Could you check a few things on this model? Use its own coordinates, in mm. A direction names the side the tool comes from. Coordinates: 2 decimals unless noted, no trailing zeros. Order: outer loops, then holes, each group sorted by start corner. A loop starts at its lowest first (then second) coordinate and runs counter-clockwise, first axis right, second up. Notation, with made-up numbers: (68, 9) - (118, 9) arc R24 ccw to (118, 44) - close; hole circle Ø3 at (17, 39). An arc over 180 degrees is marked (long way). Answer as a JSON object with one key per item and string values. Group by question number.
(1) Imagine slicing it at D-D, the plane x = 2.25. Write out the boundary of the cut face in (y, z), and give its area (3 significant figures).
(2) Please list where these lines run through material, in increasing order: probe 1 along Y at (x, z) = (8, 0); probe 2 along Z at (x, y) = (4, 0.2); probe 3 along X at (y, z) = (-0.85, 1.15).
(3) Imagine slicing it at C-C, the plane x = 0.75. Write out the boundary of the cut face in (y, z), and give its area (3 significant figures).
(4) Will these pins go through, and if not, where does the flat tip stop? P1, Ø0.5, axis at x = -1, y = 0, coming from the -Z side; P2, Ø1, axis at x = 1, y = 1, coming from the -Z side; P3, Ø1.5, axis at y = 0, z = 0.5, coming from the -X side; P4, Ø2, axis at x = 8.5, y = -1, coming from the +Z side.
(5) Which directions (+Z, -Z, +X, -X, +Y, -Y) give clear straight access to the entire face, cutting with the end or side of a thin tool? Please do faces 1 (the cylindrical face through (0.61, 0.81, 0.34)), 2 (the cylindrical face through (6, 0, 1)).
(6) Imagine slicing it at A-A, the plane y = 0. Write out the boundary of the cut face in (x, z).
(7) We'd pull the mould along Y, two halves only. Please class faces 3 (the conical face through (-0.689, -0.42, 1.894)), 4 (the flat face through (-0.8, 0, 0)), 5 (the flat face through (11, 0, 0)): pulls with the +Y half, pulls with the -Y half, needs draft (parallel to the pull), parting line crosses it, or undercut.
from build123d import *

# Parameters (mm, degrees)
CUT_EXTRUDE1_DEPTH = 0.8


with BuildPart() as part:
    # Sketch1 → Revolve1 (revolve)
    with BuildSketch(Plane.XY):
        with BuildLine():
            Line((-0.963195994, 1.91573127), (0, 2))
            Line((0, 2), (0, 0.87725))
            Line((0, 0.87725), (1.1, 0.87725))
            Line((1.1, 0.87725), (1.8, 1))
            Line((1.8, 1), (11, 1))
            Line((11, 1), (11, 0))
            Line((11, 0), (-1.6, 0))
            ThreePointArc((-1.6, 0), (-1.436628655, 1.009399034), (-0.963195994, 1.91573127))
        make_face()
    revolve(axis=Axis((11, 0, 0), (-1, 0, 0)))

    # Sketch2 → Revolve2 (revolve)
    with BuildSketch(Plane.XY):
        with BuildLine():
            Line((-0.1, 0.77725), (1.1, 0.77725))
            Line((1.1, 0.77725), (1.1, 0.87725))
            Line((1.1, 0.87725), (0.1, 0.87725))
            ThreePointArc((0.1, 0.87725), (0.029289322, 0.906539322), (0, 0.97725))
            Line((0, 0.97725), (-0.1, 0.97725))
            Line((-0.1, 0.97725), (-0.1, 0.77725))
        make_face()
    revolve(axis=Axis((1.1, 0, 0), (-1, 0, 0)))

    # Sketch3 → Cut-Extrude1 (cut)
    with BuildSketch(Plane(origin=(-1.6, 0, 0), x_dir=(0, 0, -1), z_dir=(1, 0, 0))):
        Polygon((-0.95, 0.2375), (-0.95, -0.2375), (-0.38, -0.187631462), (-0.2375, -0.2375), (-0.187631462, -0.38), (-0.2375, -0.95), (0.2375, -0.95), (0.187631462, -0.38), (0.2375, -0.2375), (0.38, -0.187631462), (0.95, -0.2375), (0.95, 0.2375), (0.38, 0.187631462), (0.2375, 0.2375), (0.187631462, 0.38), (0.2375, 0.95), (-0.2375, 0.95), (-0.187631462, 0.38), (-0.2375, 0.2375), (-0.38, 0.187631462), align=None)
    extrude(amount=CUT_EXTRUDE1_DEPTH, mode=Mode.SUBTRACT)


solid = part.part
Result set:
{
 "1": {"outline": "circle Ø2 at (0, 0)", "area": "3.14 mm^2"},
 "2": {"probe 1": "y = -1 to 1", "probe 2": "z = -0.98 to 0.98", "probe 3": "x = -1.26 to 0"},
 "3": {"outline": "circle Ø1.75 at (0, 0)", "area": "2.42 mm^2"},
 "4": {"P1": "stops at z = -1.93", "P2": "stops at z = -0.72", "P3": "stops at x = -1.58", "P4": "stops at z = 1"},
 "5": {"face 1": "none", "face 2": "+X"},
 "6": {"outline": "(-1.46, -0.95) arc R3.2 ccw to (-0.96, -1.92) - (0, -2) - (0, -0.98) arc R0.1 cw to (0.1, -0.88) - (1.1, -0.88) - (1.8, -1) - (11, -1) - (11, 1) - (1.8, 1) - (1.1, 0.88) - (0.1, 0.88) arc R0.1 cw to (0, 0.98) - (0, 2) - (-0.96, 1.92) arc R3.2 ccw to (-1.46, 0.95) - (-0.8, 0.95) - (-0.8, -0.95) - close"},
 "7": {"face 3": "parting line crosses it", "face 4": "undercut", "face 5": "needs draft"}
}
